Design review of the part shown in the three views and the two pictorial views. Dimensions are in mm from the part's minimum x, y and z. Give positions to 0.01 mm unless a question says otherwise; leave off trailing zeros. Loops run counter-clockwise (first coordinate to the right, second up) from the corner with the lowest first, then second, coordinate; pieces in that order, holes last. Notation, with made-up numbers: (66, 51.25) -> (102, 51.25) arc R23 ccw to (102, 68.25) -> close; hole circle Ø10 at (73.5, -16). An arc over 180 degrees is marked (long way). Answer as CSV lines item,"result".
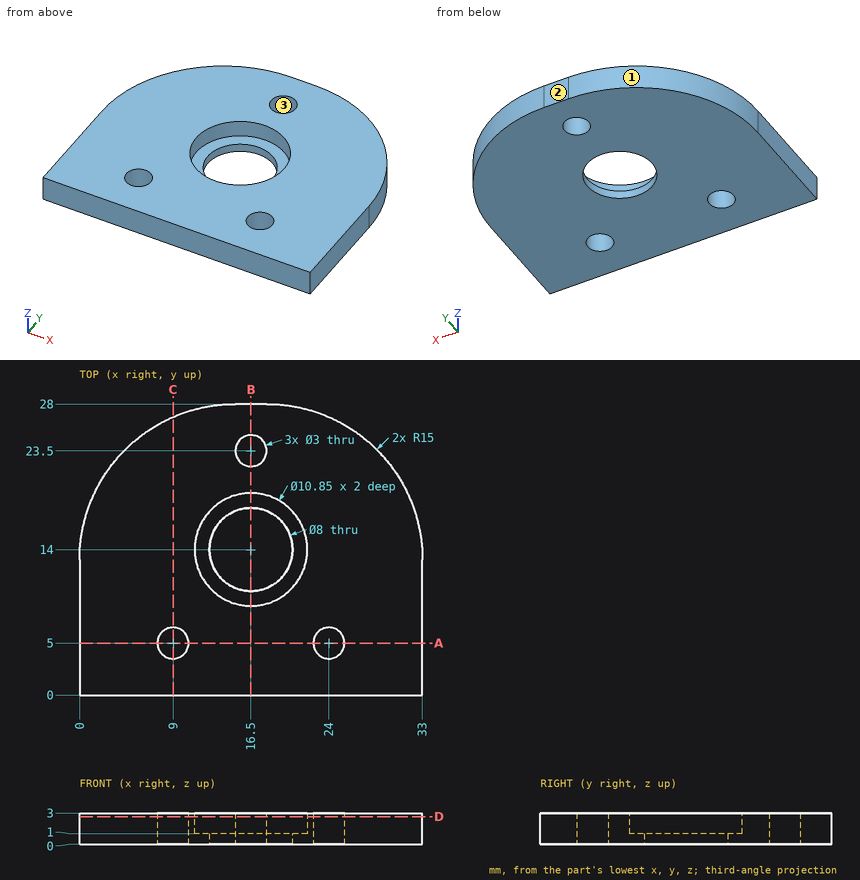
Q1. To check wall thickness, follow probe 1 along Y at (x, z) = (16.5, 0.7); probe 2 along Y at (x, z) = (16.5, 2.45) (3 decimals); probe 3 along Y at (x, z) = (30, 0.8). State the ranges of each line that lie inside material, in increasing order. Write a range as from..to.
Filled sheet:
probe 1,"y = 0..10, 18..22, 25..28"
probe 2,"y = 0..8.575, 19.425..22, 25..28"
probe 3,"y = 0..22"
Q2. We need section B-B, the plane x = 16.5. State the section outline as (y, z) points (3 decimals), and give its area (3 significant figures).
Filled sheet:
outline,"(0, 0) -> (10, 0) -> (10, 1) -> (8.575, 1) -> (8.575, 3) -> (0, 3) -> close; (18, 0) -> (22, 0) -> (22, 3) -> (19.425, 3) -> (19.425, 1) -> (18, 1) -> close; (25, 0) -> (28, 0) -> (28, 3) -> (25, 3) -> close"
area,"45.3 mm^2"
Q3. The part is to be moulded in two halves that separate along X. For the marked faces 1, 2 and 3, say which applies: pulls with the +X half, pulls with the -X half, needs draft (parallel to the pull), parting line crosses it, or undercut.
Filled sheet:
face 1,"pulls with the -X half"
face 2,"needs draft"
face 3,"undercut"
Q4. Clearance check with flat-ended pins moving along their axes: pin 1 Ø4 at (x, y) = (9, 21.5) entering from -Z; pin 2 Ø6.5 at (x, y) = (16.5, 14) entering from -Z; pin 3 Ø10 at (x, y) = (16.5, 14) entering from +Z. State where each tip first meets the part, or that it passes through.
Filled sheet:
pin 1,"stops at z = 0"
pin 2,"passes through"
pin 3,"stops at z = 1"
Q5. We need section A-A, the plane y = 5. State the section outline as (x, z) points.
Filled sheet:
outline,"(0, 0) -> (7.5, 0) -> (7.5, 3) -> (0, 3) -> close; (10.5, 0) -> (22.5, 0) -> (22.5, 3) -> (10.5, 3) -> close; (25.5, 0) -> (33, 0) -> (33, 3) -> (25.5, 3) -> close"
Q6. We need section D-D, the plane z = 2.65. State the section outline as (x, y) points (3 decimals).
Filled sheet:
outline,"(0, 0) -> (33, 0) -> (33, 13) arc R15 ccw to (18, 28) -> (15, 28) arc R15 ccw to (0, 13) -> close; hole circle Ø3 at (9, 5); hole circle Ø10.85 at (16.5, 14); hole circle Ø3 at (16.5, 23.5); hole circle Ø3 at (24, 5)"
Q7. We need section C-C, the plane x = 9. State the section outline as (y, z) points.
Filled sheet:
outline,"(0, 0) -> (3.5, 0) -> (3.5, 3) -> (0, 3) -> close; (6.5, 0) -> (26.75, 0) -> (26.75, 3) -> (6.5, 3) -> close"
